```python
from build123d import *

# Parameters (mm, degrees)
BOSS_EXTRUDE4_DEPTH = 45
SHELL3_T            = -5
BOSS_EXTRUDE5_START = -5
BOSS_EXTRUDE5_DEPTH = 5
SKETCH10_R          = 31.25
SKETCH10_R_2        = 21.25
SKETCH10_R_3        = 21
SKETCH10_R_4        = 11
BOSS_EXTRUDE6_DEPTH = 12
FILLET2_R           = 5
CHAMFER1_SIZE       = 1


with BuildPart() as part:
    # Sketch8 → Boss-Extrude4 (new body)
    with BuildSketch(Plane.XY):
        with BuildLine():
            Line((2.09348148, 59.963466672), (73.308425925, 57.47716667))
            ThreePointArc((73.308425925, 57.47716667), (108.131921611, 30.036644892), (92.450170063, -11.433112229))
            Line((92.450170063, -11.433112229), (32.720272102, -50.292979566))
            ThreePointArc((32.720272102, -50.292979566), (-57.811074578, -16.058631827), (2.09348148, 59.963466672))
        make_face()
    extrude(amount=BOSS_EXTRUDE4_DEPTH)

    # Shell3
    shell3_openings = [part.faces().sort_by_distance(p)[0] for p in [
        (19.954889275, 5.543024799, 45),
    ]]
    offset(amount=SHELL3_T, openings=shell3_openings, kind=Kind.INTERSECTION)

    # Sketch9 → Boss-Extrude5 (add)
    with BuildSketch(Plane.XY.offset(45).offset(BOSS_EXTRUDE5_START)):
        with BuildLine():
            Line((73.657339505, 67.471077782), (2.44239506, 69.957377784))
            ThreePointArc((2.44239506, 69.957377784), (-67.446253674, -18.735070465), (38.173650785, -58.675142827))
            Line((38.173650785, -58.675142827), (97.903548747, -19.81527549))
            ThreePointArc((97.903548747, -19.81527549), (117.767100707, 32.71308353), (73.657339505, 67.471077782))
        make_face()
        with BuildLine():
            Line((32.720272102, -50.292979566), (92.450170063, -11.433112229))
            ThreePointArc((92.450170063, -11.433112229), (108.131921611, 30.036644892), (73.308425925, 57.47716667))
            Line((73.308425925, 57.47716667), (2.09348148, 59.963466672))
            ThreePointArc((2.09348148, 59.963466672), (-57.811074578, -16.058631827), (32.720272102, -50.292979566))
        make_face(mode=Mode.SUBTRACT)
    extrude(amount=BOSS_EXTRUDE5_DEPTH)

    # Sketch10 → Boss-Extrude6 (add)
    # profile 1 of 2: a face of its own
    with BuildSketch(Plane(origin=(0, 0, 5), x_dir=(-1, 0, 0), z_dir=(0, 0, -1))):
        Circle(SKETCH10_R)
        Circle(SKETCH10_R_2, mode=Mode.SUBTRACT)
    # profile 2 of 2: a face of its own
    with BuildSketch(Plane(origin=(0, 0, 5), x_dir=(-1, 0, 0), z_dir=(0, 0, -1))):
        with Locations((-72, 20)):
            Circle(SKETCH10_R_3)
        with Locations((-72, 20)):
            Circle(SKETCH10_R_4, mode=Mode.SUBTRACT)
    extrude(amount=-BOSS_EXTRUDE6_DEPTH)

    # Fillet2
    fillet2_edges = [part.edges().sort_by_distance(p)[0] for p in [
        (-52.99348503, -14.720412508, 5),
        (59.858531741, -26.671964267, 5),
        (103.314332063, 28.698425573, 5),
        (37.526496913, 53.723361115, 5),
        (31.25, 0, 5),
    ]]
    fillet(fillet2_edges, radius=FILLET2_R)

    # Chamfer1
    chamfer1_edges = [part.edges().sort_by_distance(p)[0] for p in [
        (21.25, 0, 17),
        (83, 20, 17),
    ]]
    chamfer(chamfer1_edges, length=CHAMFER1_SIZE)


solid = part.part
```
Check sheet for the modelled part. Datum: model origin and axes. Units: mm. A direction names the side the tool comes from. Give positions to 0.01 mm unless a question says otherwise; leave off trailing zeros. Write each loop counter-clockwise with the first axis right and the second up, starting at its lowest first coordinate (ties: lowest second). Pieces come first, ordered by that corner, then holes. Notation, with made-up numbers: (53, -30) - (111, -30) arc R19 cw to (111, -7) - close; hole circle Ø1 at (73, 39.5). An arc over 180 degrees is marked (long way). Answer as a JSON object with one key per item and string values. Group by question number.
1) Access from +Z, -Z, +X, -X, +Y, -Y to the whole of each face (thin tool, end or side, straight path). Record for faces 1 (the face through (37.98, 52.28, 6.5)), 2 (the face through (107.95, 30.67, 19.72)), 3 (the face through (63.003, -30.591, 19.72)), 4 (the face through (26, 1, 0)).
2) Thickness scan on probe 1 along Y at (x, z) = (0, 13); probe 2 along Y at (x, z) = (0, 43.5); probe 3 along X at (y, z) = (4, 7.5). Record the ranges inside material, lowest first. Write a range as from..to.
3) Release check for a two-part mould opening along Y. For faces 5 (the face through (38.3, -41.2, 45)), 6 (the face through (83, 20, 10)), 7 (the face through (-57.37, -17.57, 19.72)) record: pulls with the +Y half, pulls with the -Y half, needs draft (parallel to the pull), parting line crosses it, or undercut.
4) Depth check by flat-ended pin: P1, Ø11, axis at x = 69.5, y = 15, coming from the +Z side; P2, Ø12, axis at y = 20.5, z = 10, coming from the +X side; P3, Ø2, axis at x = 20, y = 35.5, coming from the +Z side. Enter the tip coordinate at first touch or a pass-through.
5) Sectioned sample at A-A (z = 14). Record the cut outline in (x, y), then the cut area to 3 significant figures.
Geometry results:
{
 "1": {"face 1": "+Z", "face 2": "-Z, +X", "face 3": "-Z, +X, -Y", "face 4": "-Z, +X, -X, +Y, -Y"},
 "2": {"probe 1": "y = -60..-55, -31.25..-21.25, 21.25..31.25, 55..60", "probe 2": "y = -70..-55, 55..70", "probe 3": "x = -59.87..-54.18, -31.67..-20.87, 20.87..31.67, 58.4..85.6, 99.52..105.92"},
 "3": {"face 5": "needs draft", "face 6": "undercut", "face 7": "parting line crosses it"},
 "4": {"P1": "stops at z = 16.09", "P2": "stops at x = 109.5", "P3": "stops at z = 5"},
 "5": {"outline": "circle Ø62.5 at (0, 0); (2.09, 59.96) arc R60 ccw (long way) to (32.72, -50.29) - (92.45, -11.43) arc R37.5 ccw to (73.31, 57.48) - close; circle Ø42 at (72, 20); hole circle Ø42.5 at (0, 0); hole (1.92, 54.97) arc R55 ccw (long way) to (29.99, -46.1) - (89.72, -7.24) arc R32.5 ccw to (73.13, 52.48) - close; hole circle Ø22 at (72, 20)", "area": "4,890 mm^2"}
}
